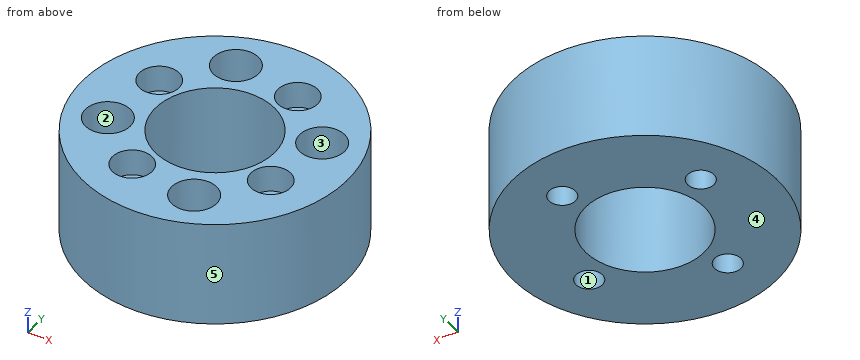
```python
from build123d import *

# Parameters (mm, degrees)
ESQUISSE1_R             = 25
ESQUISSE1_R_2           = 11.25
BOSS_EXTRU_1_DEPTH      = 20
ESQUISSE2_R             = 2.5
ENL_V_MAT_EXTRU_1_DEPTH = 41.620192023
ESQUISSE4_R             = 3.75
ENL_V_MAT_EXTRU_2_DEPTH = 5
ESQUISSE12_R            = 4.25
ENL_V_MAT_EXTRU_6_DEPTH = 7.5


with BuildPart() as part:
    # Esquisse1 → Boss.-Extru.1 (new body)
    with BuildSketch(Plane.XY):
        Circle(ESQUISSE1_R)
        Circle(ESQUISSE1_R_2, mode=Mode.SUBTRACT)
    extrude(amount=BOSS_EXTRU_1_DEPTH)

    # Esquisse2 → Enlèv. mat.-Extru.1 (cut, through all)
    with BuildSketch(Plane.XY.offset(20)):
        with Locations((-14.713385832, 6.286197369)):
            Circle(ESQUISSE2_R)
        with Locations((6.28955657, 14.711950182)):
            Circle(ESQUISSE2_R)
        with Locations((14.713385832, -6.286197369)):
            Circle(ESQUISSE2_R)
        with Locations((-6.28955657, -14.711950182)):
            Circle(ESQUISSE2_R)
    extrude(amount=-ENL_V_MAT_EXTRU_1_DEPTH, mode=Mode.SUBTRACT)

    # Esquisse4 → Enlèv. mat.-Extru.2 (cut)
    with BuildSketch(Plane.XY.offset(20)):
        with Locations((-6.28955657, -14.711950182)):
            Circle(ESQUISSE4_R)
        with Locations((14.713385832, -6.286197369)):
            Circle(ESQUISSE4_R)
        with Locations((6.28955657, 14.711950182)):
            Circle(ESQUISSE4_R)
        with Locations((-14.713385832, 6.286197369)):
            Circle(ESQUISSE4_R)
    extrude(amount=-ENL_V_MAT_EXTRU_2_DEPTH, mode=Mode.SUBTRACT)

    # Esquisse12 → Enlèv. mat.-Extru.6 (cut)
    with BuildSketch(Plane.XY.offset(20)):
        with Locations((16.24178047, 6.515716934)):
            Circle(ESQUISSE12_R)
        with Locations((-16.24178047, -6.515716934)):
            Circle(ESQUISSE12_R)
        with Locations((6.515716934, -16.24178047)):
            Circle(ESQUISSE12_R)
        with Locations((-6.515716934, 16.24178047)):
            Circle(ESQUISSE12_R)
    extrude(amount=-ENL_V_MAT_EXTRU_6_DEPTH, mode=Mode.SUBTRACT)


solid = part.part
```
CAD build for the part. Positions are in the model's coordinates, mm. Face numbers are marked on the shaded views. A direction names the side the tool comes from. Round coordinates to 2 decimals unless told otherwise and drop trailing zeros. Write each loop counter-clockwise with the first axis right and the second up, starting at its lowest first coordinate (ties: lowest second). Pieces come first, ordered by that corner, then holes. Notation, with made-up numbers: (84.25, 64.5) -> (123.25, 64.5) arc R23 ccw to (123.25, 80.5) -> close; hole circle Ø11 at (63, -16). An arc over 180 degrees is marked (long way). Answer in a Markdown table with one row per item. Add a question column.
Item 1: Saw through at A-A, the plane y = 0. Write the cut outline in (x, z).
Item 2: Saw through at D-D, the plane y = -19.5. Write the cut outline in (x, z), then the cut area to 3 significant figures.
Item 3: Which spindle directions (+Z, -Z, +X, -X, +Y, -Y) get a long thin tool onto all of the face, cutting with end or side? Do the marked faces 1 and 2. Say none if no direction does.
Item 4: Saw through at C-C, the plane z = 6.75. Write the cut outline in (x, y), then the cut area to 3 significant figures.
Item 5: Mould opens along Y. For the marked faces 3, 4 and 5 say: pulls with the +Y half, pulls with the -Y half, needs draft (parallel to the pull), parting line crosses it, or undercut.
Item 6: Drop flat-ended pins along their axis: pin 1 Ø4 at (x, y) = (5.5, 14.5) entering from +Z; pin 2 Ø4.5 at (x, y) = (14.71, -6.29) entering from +Z; pin 3 Ø5 at (x, z) = (-4, 12.5) entering from +Y; pin 4 Ø4 at (y, z) = (-4.5, 6.5) entering from -X. Give the stop position or say it passes through.
Item 7: Drill centre lines: line 1 (Y direction, x = -0.5, z = 13.5) (3 decimals); line 2 (Y direction, x = 5.5, z = 4); line 3 (Z direction, x = -19, y = -6). Where is each one in solid material? Low to high. Write a range as from..to.
Findings below:
| question | item | result |
|---|---|---|
| 1 | outline | (-25, 0) -> (-11.25, 0) -> (-11.25, 20) -> (-25, 20) -> close; (11.25, 0) -> (25, 0) -> (25, 20) -> (11.25, 20) -> close |
| 2 | outline | (-15.64, 0) -> (15.64, 0) -> (15.64, 20) -> (9.24, 20) -> (9.24, 12.5) -> (3.79, 12.5) -> (3.79, 20) -> (-15.64, 20) -> close |
| 2 | area | 585 mm^2 |
| 3 | face 1 | +Z, -Z |
| 3 | face 2 | +Z |
| 4 | outline | circle Ø50 at (0, 0); hole circle Ø5 at (-14.71, 6.29); hole circle Ø22.5 at (0, 0); hole circle Ø5 at (-6.29, -14.71); hole circle Ø5 at (6.29, 14.71); hole circle Ø5 at (14.71, -6.29) |
| 4 | area | 1,490 mm^2 |
| 5 | face 3 | undercut |
| 5 | face 4 | needs draft |
| 5 | face 5 | parting line crosses it |
| 6 | pin 1 | stops at z = 15 |
| 6 | pin 2 | passes through |
| 6 | pin 3 | stops at y = 24.95 |
| 6 | pin 4 | stops at x = -24.87 |
| 7 | line 1 | y = -24.995..-11.239, 11.239..24.995 |
| 7 | line 2 | y = -24.39..-9.81, 9.81..12.34, 17.08..24.39 |
| 7 | line 3 | z = 0..12.5 |
